The model under review builds one solid part; all positions refer to its coordinate system, in mm. Coordinates: 2 decimals unless noted, no trailing zeros. Order: outer loops, then holes, each group sorted by start corner. A loop starts at its lowest first (then second) coordinate and runs counter-clockwise, first axis right, second up.
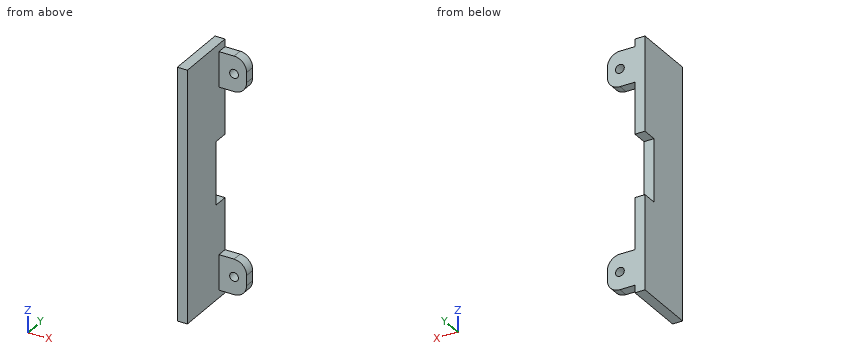
```python
from build123d import *

# Parameters (mm, degrees)
RESSALTO_EXTRUS_O1_DEPTH = 100
ESBO_O2_R                = 1.75
ESBO_O2_W                = 11
ESBO_O2_H                = 3
ESBO_O2_H_2              = 66
CORTE_EXTRUS_O1_DEPTH    = 100
FILETE1_R                = 5
ESBO_O3_W                = 25
ESBO_O3_H                = 12
CORTE_EXTRUS_O2_DEPTH    = 100


with BuildPart() as part:
    # Esboço1 → Ressalto-extrusão1 (new body)
    with BuildSketch(Plane.XY):
        Polygon((15, 0), (0, 0), (0, -25), (4, -25), (4, -4), (15, -4), align=None)
    extrude(amount=RESSALTO_EXTRUS_O1_DEPTH)

    # Esboço2 → Corte-extrusão1 (cut)
    with BuildSketch(Plane(origin=(0, 0, 0), x_dir=(1, 0, 0), z_dir=(0, 1, 0))):
        with Locations((10, -10)):
            Circle(ESBO_O2_R)
        with Locations((10, -90)):
            Circle(ESBO_O2_R)
        with Locations((9.5, -1.5)):
            Rectangle(ESBO_O2_W, ESBO_O2_H)
        with Locations((9.5, -50)):
            Rectangle(ESBO_O2_W, ESBO_O2_H_2)
        with Locations((9.5, -98.5)):
            Rectangle(ESBO_O2_W, ESBO_O2_H)
    extrude(amount=-CORTE_EXTRUS_O1_DEPTH, mode=Mode.SUBTRACT)

    # Filete1
    filete1_edges = [part.edges().sort_by_distance(p)[0] for p in [
        (15, -2, 97),
        (15, -2, 3),
        (15, -2, 17),
        (15, -2, 83),
    ]]
    fillet(filete1_edges, radius=FILETE1_R)

    # Esboço3 → Corte-extrusão2 (cut)
    with BuildSketch(Plane.ZY):
        with Locations((50, 0)):
            Rectangle(ESBO_O3_W, ESBO_O3_H)
    extrude(amount=-CORTE_EXTRUS_O2_DEPTH, mode=Mode.SUBTRACT)


solid = part.part
```
(1) We need section A-A, the plane y = -5. Write out the cut boundary in (x, z), and give its area (3 significant figures).
A:
outline: (0, 0) - (4, 0) - (4, 37.5) - (0, 37.5) - close; (0, 62.5) - (4, 62.5) - (4, 100) - (0, 100) - close
area: 300 mm2
(2) Wall thickness on probe 1 along Z at (x, y) = (10, -0.95); probe 2 along X at (y, z) = (-1.05, 10); probe 3 along X at (y, z) = (-11.25, 47): over which ranges is each line inside the solid? List them lowest first.
A:
probe 1: z = 3 to 8.25, 11.75 to 17, 83 to 88.25, 91.75 to 97
probe 2: x = 0 to 8.25, 11.75 to 15
probe 3: x = 0 to 4
(3) We need section B-B, the plane z = 90. Write out the cut boundary in (x, y), and give its area (3 significant figures).
A:
outline: (0, -25) - (4, -25) - (4, -4) - (8.25, -4) - (8.25, 0) - (0, 0) - close; (11.75, -4) - (15, -4) - (15, 0) - (11.75, 0) - close
area: 130 mm2
(4) We need section C-C, the plane x = 5.5. Write out the cut boundary in (y, z), and give its area (3 significant figures).
A:
outline: (-4, 3) - (0, 3) - (0, 17) - (-4, 17) - close; (-4, 83) - (0, 83) - (0, 97) - (-4, 97) - close
area: 112 mm2
(5) For pin 1 Ø1.5 at (y, z) = (-19, 21) entering from +X; pin 2 Ø1.2 at (x, y) = (7.5, -1.5) entering from -Z; pin 3 Ø1.2 at (x, y) = (6.5, -2) entering from +Z; pin 4 Ø6 at (x, y) = (12.5, -7.5) entering from +Z, all flat-tipped, find the tip position at first contact; note any pin that passes through.
A:
pin 1: stops at x = 4
pin 2: stops at z = 3
pin 3: stops at z = 97
pin 4: passes through
(6) We need section D-D, the plane z = 22. Write out the cut boundary in (x, y), and give its area (3 significant figures).
A:
outline: (0, -25) - (4, -25) - (4, 0) - (0, 0) - close
area: 100 mm2
